from build123d import *

# Parameters (mm, degrees)
F1_DEPTH = 50.8
F2_R     = 9.52499
F4_DEPTH = 44.45
F6_DEPTH = 6.35


# Not quite as in the source:
# - a fillet or chamfer is up to 0.001 mm smaller than in the source, because OpenCascade refuses the exact size


with BuildPart() as f1:
    # F0 (on Right) → F1 (new body)
    with BuildSketch(Plane.YZ):
        with BuildLine():
            Line((9.525, 0), (-9.525, 0))
            ThreePointArc((-9.525, 0), (0, -9.525), (9.525, 0))
        make_face()
    extrude(amount=F1_DEPTH)

    # F2 (radius 9.525 in the source; OpenCascade refuses exactly that, so slightly less here)
    f2_edges = [f1.edges().sort_by_distance(p)[0] for p in [
        (0, 0, -9.525),
    ]]
    fillet(f2_edges, radius=F2_R)

    # F3 (on face) → F4 (cut)
    with BuildSketch(Plane.YZ.offset(50.8)):
        with BuildLine():
            Line((6.35, 0), (-6.35, 0))
            ThreePointArc((-6.35, 0), (0, -6.35), (6.35, 0))
        make_face()
    extrude(amount=-F4_DEPTH, mode=Mode.SUBTRACT)

    # F5 (on face) → F6 (cut)
    with BuildSketch(Plane.YZ.offset(6.35)):
        with BuildLine():
            Line((3.175, 0), (-3.175, 0))
            Line((-3.175, 0), (-3.175, -5.499261314))
            ThreePointArc((-3.175, -5.499261314), (0, -6.35), (3.175, -5.499261314))
            Line((3.175, -5.499261314), (3.175, 0))
        make_face()
    extrude(amount=-F6_DEPTH, mode=Mode.SUBTRACT)


solid = f1.part
Read the model definition and answer for the solid it produces. Units are mm, in the model's axes. A direction names the side the tool comes from. Give positions to 0.01 mm unless a question says otherwise; leave off trailing zeros. Write each loop counter-clockwise with the first axis right and the second up, starting at its lowest first coordinate (ties: lowest second). Pieces come first, ordered by that corner, then holes. Notation, with made-up numbers: M -19,80 L -3,80 A31 ccw -3,114 Z; hole C -14.75,56 d10. An arc over 180 degrees is marked long. One line per item, written item: value. Start each with the question number.
(1) Find section A-A (x = 24). Determine the outline of the cut face in (y, z) (3 decimals), plus the area to 3 significant figures.
(2) Determine the mould class of faces 4 (the flat face through (6.35, 4, -2)), 5 (the cylindrical face through (29.874, -0.209, -9.523)), 6 (the flat face through (25, -8, 0)) for opening direction Y: pulls with the +Y half, pulls with the -Y half, needs draft (parallel to the pull), parting line crosses it, or undercut.
(3) Find the intervals of material crossed by line 1 (Y direction, x = 12, z = -0.75); line 2 (Y direction, x = 9, z = -5); line 3 (Z direction, x = 42.5, y = 7.25), in increasing order.
(4) Flat-ended cylindrical pins translate along their axes: pin 1 Ø1.5 at (x, y) = (8, -4) entering from -Z; pin 2 Ø3.5 at (y, z) = (-4, -1.5) entering from +X; pin 3 Ø1 at (x, z) = (38, -7.5) entering from +Y. Find the tip coordinate at first contact, or state that the pin passes through.
(5) A tool of negligible diameter and unlimited length cuts with its end or side. For faces 1 (the flat face through (50.8, 0, -7)), 2 (the flat face through (6.35, -4, -2)), 3 (the flat face through (3, -3.175, -3)), from which of +Z, -Z, +X, -X, +Y, -Y can it reach the whole face along a straight path? Write none if from no direction.
Results below:
1. outline: M -9.525,0 A9.525 ccw 9.525,0 L 6.35,0 A6.35 cw -6.35,0 Z
1. area: 79.2 mm^2
2. face 4: undercut
2. face 5: parting line crosses it
2. face 6: needs draft
3. line 1: y = -9.5 to -6.31, 6.31 to 9.5
3. line 2: y = -8.09 to -3.91, 3.91 to 8.09
3. line 3: z = -6.18 to 0
4. pin 1: stops at z = -8.85
4. pin 2: stops at x = 6.35
4. pin 3: stops at y = 6.46
5. face 1: +Z, -Z, +X, +Y, -Y
5. face 2: +Z, +X
5. face 3: +Z, +X, -X
